```python
from build123d import *

# Parameters (mm, degrees)
SKETCH1_W           = 1300
SKETCH1_H           = 600
SKETCH1_W_2         = 1117.676372874
SKETCH1_H_2         = 40
BOSS_EXTRUDE1_DEPTH = 20
SKETCH2_W           = 40
SKETCH2_H           = 10
BOSS_EXTRUDE2_DEPTH = 40
SKETCH3_R           = 5
CUT_EXTRUDE1_DEPTH  = 10
SKETCH4_W           = 40
SKETCH4_H           = 10
BOSS_EXTRUDE3_DEPTH = 50
SKETCH5_R           = 5
CUT_EXTRUDE2_DEPTH  = 10
FILLET1_R           = 10
FILLET2_R           = 10
FILLET3_R           = 10
FILLET4_R           = 10
FILLET5_R           = 10
FILLET6_R           = 10
FILLET7_R           = 10
FILLET8_R           = 10
SKETCH6_W           = 20
SKETCH6_H           = 40
BOSS_EXTRUDE4_DEPTH = 260
SKETCH7_W           = 20
SKETCH7_H           = 40
BOSS_EXTRUDE5_DEPTH = 35
SKETCH8_W           = 20
SKETCH8_H           = 600
CUT_EXTRUDE3_DEPTH  = 100
SKETCH9_W           = 20
SKETCH9_H           = 600
CUT_EXTRUDE4_DEPTH  = 300
SKETCH10_W          = 32
SKETCH10_H          = 32
SKETCH10_W_2        = 26
SKETCH10_H_2        = 26
BOSS_EXTRUDE6_DEPTH = 130


with BuildPart() as part:
    # Sketch1 → Boss-Extrude1 (new body)
    with BuildSketch(Plane.XY):
        Rectangle(SKETCH1_W, SKETCH1_H)
        Rectangle(SKETCH1_W_2, SKETCH1_H_2, mode=Mode.SUBTRACT)
    extrude(amount=BOSS_EXTRUDE1_DEPTH)

    # Sketch2 → Boss-Extrude2 (add)
    with BuildSketch(Plane.XY.offset(20)):
        with Locations((-338.838186437, 25)):
            Rectangle(SKETCH2_W, SKETCH2_H)
        with Locations((-338.838186437, -25)):
            Rectangle(SKETCH2_W, SKETCH2_H)
    extrude(amount=BOSS_EXTRUDE2_DEPTH)

    # Sketch3 → Cut-Extrude1 (cut)
    with BuildSketch(Plane.XZ.offset(30)):
        with Locations((-338.838186437, 40)):
            Circle(SKETCH3_R)
    extrude(amount=-CUT_EXTRUDE1_DEPTH, mode=Mode.SUBTRACT)

    # Sketch4 → Boss-Extrude3 (add)
    with BuildSketch(Plane.XY.offset(60)):
        with Locations((-338.838186437, 25)):
            Rectangle(SKETCH4_W, SKETCH4_H)
    extrude(amount=BOSS_EXTRUDE3_DEPTH)

    # Sketch5 → Cut-Extrude2 (cut)
    with BuildSketch(Plane.XZ.offset(-20)):
        with Locations(Location((-338.838186437, 90, 0), (0, 0, 270))):
            Circle(SKETCH5_R)
    extrude(amount=-CUT_EXTRUDE2_DEPTH, mode=Mode.SUBTRACT)

    # Fillet1
    fillet1_edges = [part.edges().sort_by_distance(p)[0] for p in [
        (-318.838186437, -25, 20),
    ]]
    fillet(fillet1_edges, radius=FILLET1_R)

    # Fillet2
    fillet2_edges = [part.edges().sort_by_distance(p)[0] for p in [
        (-318.838186437, 25, 20),
    ]]
    fillet(fillet2_edges, radius=FILLET2_R)

    # Fillet3
    fillet3_edges = [part.edges().sort_by_distance(p)[0] for p in [
        (-358.838186437, -25, 20),
    ]]
    fillet(fillet3_edges, radius=FILLET3_R)

    # Fillet4
    fillet4_edges = [part.edges().sort_by_distance(p)[0] for p in [
        (-358.838186437, 25, 20),
    ]]
    fillet(fillet4_edges, radius=FILLET4_R)

    # Fillet5
    fillet5_edges = [part.edges().sort_by_distance(p)[0] for p in [
        (-318.838186437, -25, 60),
    ]]
    fillet(fillet5_edges, radius=FILLET5_R)

    # Fillet6
    fillet6_edges = [part.edges().sort_by_distance(p)[0] for p in [
        (-358.838186437, -25, 60),
    ]]
    fillet(fillet6_edges, radius=FILLET6_R)

    # Fillet7
    fillet7_edges = [part.edges().sort_by_distance(p)[0] for p in [
        (-358.838186437, 25, 110),
    ]]
    fillet(fillet7_edges, radius=FILLET7_R)

    # Fillet8
    fillet8_edges = [part.edges().sort_by_distance(p)[0] for p in [
        (-318.838186437, 25, 110),
    ]]
    fillet(fillet8_edges, radius=FILLET8_R)

    # Sketch6 → Boss-Extrude4 (add)
    with BuildSketch(Plane.ZY.offset(-558.838186437)):
        with Locations((10, 0)):
            Rectangle(SKETCH6_W, SKETCH6_H)
    extrude(amount=BOSS_EXTRUDE4_DEPTH)

    # Sketch7 → Boss-Extrude5 (add)
    with BuildSketch(Plane(origin=(-558.838186437, 0, 0), x_dir=(0, 0, -1), z_dir=(1, 0, 0))):
        with Locations((-10, 0)):
            Rectangle(SKETCH7_W, SKETCH7_H)
    extrude(amount=BOSS_EXTRUDE5_DEPTH)

    # Sketch8 → Cut-Extrude3 (cut)
    with BuildSketch(Plane.ZY.offset(650)):
        with Locations((10, 0)):
            Rectangle(SKETCH8_W, SKETCH8_H)
    extrude(amount=-CUT_EXTRUDE3_DEPTH, mode=Mode.SUBTRACT)

    # Sketch9 → Cut-Extrude4 (cut)
    with BuildSketch(Plane(origin=(650, 0, 0), x_dir=(0, 0, -1), z_dir=(1, 0, 0))):
        with Locations((-10, 0)):
            Rectangle(SKETCH9_W, SKETCH9_H)
    extrude(amount=-CUT_EXTRUDE4_DEPTH, mode=Mode.SUBTRACT)

    # Sketch10 → Boss-Extrude6 (add)
    # profile 1 of 4: a face of its own
    with BuildSketch(Plane(origin=(0, 0, 0), x_dir=(-1, 0, 0), z_dir=(0, 0, -1))):
        with Locations((511, -261)):
            Rectangle(SKETCH10_W, SKETCH10_H)
        with Locations((511, -261)):
            Rectangle(SKETCH10_W_2, SKETCH10_H_2, mode=Mode.SUBTRACT)
    # profile 2 of 4: a face of its own
    with BuildSketch(Plane(origin=(0, 0, 0), x_dir=(-1, 0, 0), z_dir=(0, 0, -1))):
        with Locations((-311, -261)):
            Rectangle(SKETCH10_W, SKETCH10_H)
        with Locations((-311, -261)):
            Rectangle(SKETCH10_W_2, SKETCH10_H_2, mode=Mode.SUBTRACT)
    # profile 3 of 4: a face of its own
    with BuildSketch(Plane(origin=(0, 0, 0), x_dir=(-1, 0, 0), z_dir=(0, 0, -1))):
        with Locations((-311, 261)):
            Rectangle(SKETCH10_W, SKETCH10_H)
        with Locations((-311, 261)):
            Rectangle(SKETCH10_W_2, SKETCH10_H_2, mode=Mode.SUBTRACT)
    # profile 4 of 4: a face of its own
    with BuildSketch(Plane(origin=(0, 0, 0), x_dir=(-1, 0, 0), z_dir=(0, 0, -1))):
        with Locations((511, 261)):
            Rectangle(SKETCH10_W, SKETCH10_H)
        with Locations((511, 261)):
            Rectangle(SKETCH10_W_2, SKETCH10_H_2, mode=Mode.SUBTRACT)
    extrude(amount=BOSS_EXTRUDE6_DEPTH)


solid = part.part
```
Source: CAD feature listing. Evaluate the final solid. Frame: model axes, mm. A direction names the side the tool comes from. Coordinates: 2 decimals unless noted, no trailing zeros. Loops run counter-clockwise (first coordinate to the right, second up) from the corner with the lowest first, then second, coordinate; pieces in that order, holes last. Notation, with made-up numbers: M 84,79 L 122,79 A32 cw 122,110 Z; hole C -30,51.5 d1. An arc over 180 degrees is marked long. Use a Markdown table: item, result. Add a question column.
Q1. Draft query along X for faces 1 (the flat face through (-497, -261, -130)), 2 (the flat face through (295, 261, -64)), 3 (the flat face through (-550, 4, 10)). Return one class per face: pulls with the +X half, pulls with the -X half, needs draft (parallel to the pull), parting line crosses it, or undercut.
Q2. Section query A-A, the plane z = -35. State how many separate pieces and enclosed holes the cut face has, and give its area (3 significant figures).
Q3. Material intervals for L1, parallel to X at y = 22.75, z = 90; L2, parallel to Y at x = 195, z = 3; L3, parallel to Z at x = -427.5, y = -227, sorted ascending.
Q4. First-contact query: pin 1 (9.5 mm diameter, centred on x = 314, z = -36.5, fed in from +Y); pin 2 (1.5 mm diameter, centred on x = -281, y = -123, fed in from +Z); pin 3 (8 mm diameter, centred on y = -258, z = -57.5, fed in from +X). Flat tips, straight axial feed; report the tip coordinate or a pass-through.
Q5. Section query B-B, the plane x = -153. Return loops of the section in (y, z), and give its area (3 significant figures).
Q6. Section query C-C, the plane y = 205. Return loops of the section in (x, z).
Q7. Access query for faces 4 (the flat face through (311, -277, -64)), 5 (the flat face through (324, -261, -64)), 6 (the flat face through (295, -261, -64)). Directions: +Z, -Z, +X, -X, +Y, -Y. A direction counts if a zero-diameter tool reaches every point of the face in a straight line with its end or side. Return the directions, or none.
Result:
| question | item | result |
|---|---|---|
| 1 | face 1 | needs draft |
| 1 | face 2 | undercut |
| 1 | face 3 | pulls with the -X half |
| 2 | separate pieces | 4 |
| 2 | enclosed holes | 4 |
| 2 | area | 1,390 mm2 |
| 3 | L1 | x = -358.84 to -343.84, -333.84 to -318.84 |
| 3 | L2 | y = -300 to -20, 20 to 300 |
| 3 | L3 | z = 0 to 20 |
| 4 | pin 1 | stops at y = 277 |
| 4 | pin 2 | stops at z = 20 |
| 4 | pin 3 | stops at x = 327 |
| 5 | outline | M -300,0 L -20,0 L -20,20 L -300,20 Z; M 20,0 L 300,0 L 300,20 L 20,20 Z |
| 5 | area | 11,200 mm2 |
| 6 | outline | M -550,0 L 350,0 L 350,20 L -550,20 Z |
| 7 | face 4 | -Z, +X, -X, -Y |
| 7 | face 5 | -Z |
| 7 | face 6 | -Z, +Y, -Y |
